Can you work these out from the drawing? Everything is in mm from the part's minimum corner. A direction names the side the tool comes from. Coordinates: 2 decimals unless noted, no trailing zeros. Loops run counter-clockwise (first coordinate to the right, second up) from the corner with the lowest first, then second, coordinate; pieces in that order, holes last. Notation, with made-up numbers: (23, 30) - (38, 30) arc R5 ccw to (38, 35) - close; hole circle Ø11 at (60, 88.25). An arc over 180 degrees is marked (long way). Put each result on its own line as item: value. Start each with the question number.
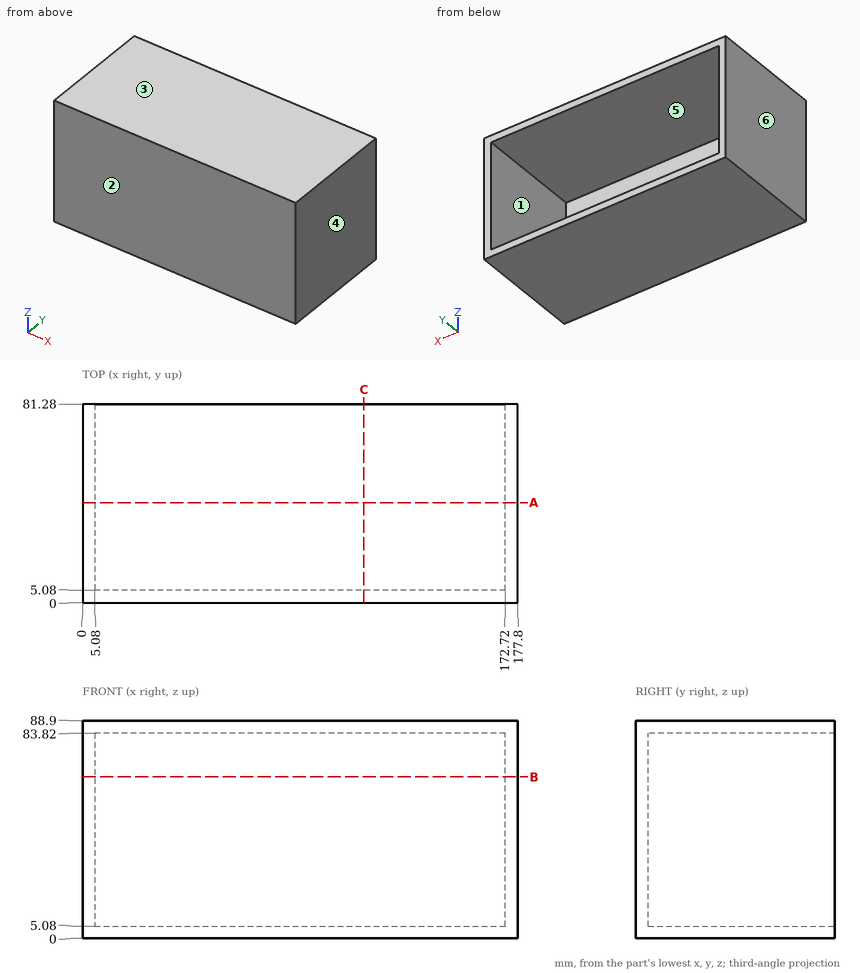
(1) I want a section at C-C on x = 115. List the corners of the cut face in (y, z) for me.
(2) If we mould it in two halves opening along X, with no side actions, what happens to the marked faces 3, 4, 5 and 6? For each: pulls with the +X half, pulls with the -X half, needs draft (parallel to the pull), parting line crosses it, or undercut.
(3) For pin 1 Ø2 at (x, z) = (88.5, 17.5) entering from +Y; pin 2 Ø1 at (y, z) = (45, 34) entering from -X, each with a flat end and sliding along its axis, tell me the tip position at first contact or that it passes through.
(4) I need wall thicknesses on L1, parallel to X at y = 9, z = 81; L2, parallel to Z at x = 145, y = 26.5; L3, parallel to Y at x = 70, z = 68.5. Which ranges of each line are inside material? Lowest first, please. Write a range as [from, to].
(5) I want a section at A-A on y = 41. List the corners of the cut face in (x, z) for me, and give its area (3 significant figures).
(6) Which directions (+Z, -Z, +X, -X, +Y, -Y) give clear straight access to the entire face, cutting with the end or side of a thin tool? Please do the marked faces 1 and 2.
(7) I want a section at B-B on z = 66. List the corners of the cut face in (x, y) for me, and give its area (3 significant figures).
Answer sheet:
1. outline: (0, 0) - (81.28, 0) - (81.28, 5.08) - (5.08, 5.08) - (5.08, 83.82) - (81.28, 83.82) - (81.28, 88.9) - (0, 88.9) - close
2. face 3: needs draft
2. face 4: pulls with the +X half
2. face 5: undercut
2. face 6: pulls with the -X half
3. pin 1: stops at y = 5.08
3. pin 2: stops at x = 0
4. L1: x = [0, 5.08], [172.72, 177.8]
4. L2: z = [0, 5.08], [83.82, 88.9]
4. L3: y = [0, 5.08]
5. outline: (0, 0) - (177.8, 0) - (177.8, 88.9) - (0, 88.9) - close; hole (5.08, 5.08) - (172.72, 5.08) - (172.72, 83.82) - (5.08, 83.82) - close
5. area: 2,610 mm^2
6. face 1: +Y
6. face 2: +Z, -Z, +X, -X, -Y
7. outline: (0, 0) - (177.8, 0) - (177.8, 81.28) - (172.72, 81.28) - (172.72, 5.08) - (5.08, 5.08) - (5.08, 81.28) - (0, 81.28) - close
7. area: 1,680 mm^2
